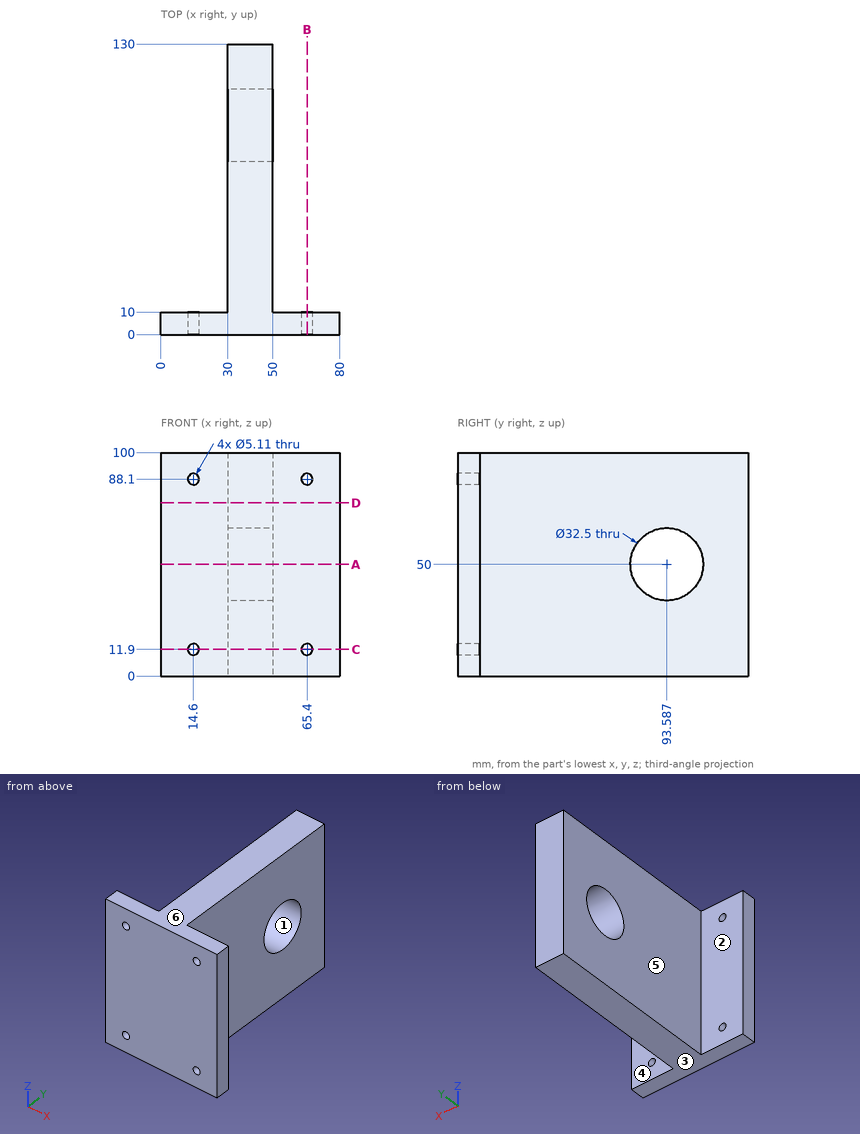
The drawing under review shows one solid part. Ordinate dimensions are in mm from its lowest x, y, z. A direction names the side the tool comes from. Round coordinates to 2 decimals unless told otherwise and drop trailing zeros. Loops run counter-clockwise (first coordinate to the right, second up) from the corner with the lowest first, then second, coordinate; pieces in that order, holes last. Notation, with made-up numbers: (81.5, 80) -> (125.5, 80) arc R11 cw to (125.5, 92) -> close; hole circle Ø8 at (29, 56). An arc over 180 degrees is marked (long way). One line per question, with ' | ' between items. Start each with the question number.
Item 1: For pin 1 (6 mm diameter, centred on y = 57, z = 31.5, fed in from +X); pin 2 (8 mm diameter, centred on x = 12.5, z = 88.5, fed in from +Y), all flat-tipped, find the tip position at first contact; note any pin that passes through.
Item 2: Add section D-D, the plane z = 77.5. Write out the cut boundary in (x, y), then the cut area to 3 significant figures.
Item 3: Wall thickness on line 1 along Z through (x, y) = (14.6, 2.25) (3 decimals); line 2 along Z through (x, y) = (65, 8); line 3 along X through (y, z) = (5, 88): over which ranges is each line inside the solid? List them lowest first. Write a range as [from, to].
Item 4: Add section A-A, the plane z = 50. Write out the cut boundary in (x, y).
Item 5: Draft analysis for pull direction Z (two halves, no side actions). For the marked faces 1, 2 and 3, state which applies: +Z half, -Z half, draft (parallel to the pull), parting line (faces both ways), or undercut.
Item 6: Machinability: for the marked faces 4, 5 and 6, which of the approach directions +Z, -Z, +X, -X, +Y, -Y give a long, thin tool a straight path to every point of the face, cutting with its end or side? Answer none if there is none.
Item 7: Add section C-C, the plane z = 11.9. Write out the cut boundary in (x, y) (3 decimals), then the cut area to 3 significant figures.
Item 8: Add section B-B, the plane x = 65.4. Write out the cut boundary in (y, z) (3 decimals).
Return value:
1) pin 1: stops at x = 50 | pin 2: stops at y = 10
2) outline: (0, 0) -> (80, 0) -> (80, 10) -> (50, 10) -> (50, 130) -> (30, 130) -> (30, 10) -> (0, 10) -> close | area: 3,200 mm2
3) line 1: z = [0, 9.345], [14.455, 85.545], [90.655, 100] | line 2: z = [0, 9.38], [14.42, 85.58], [90.62, 100] | line 3: x = [0, 12.05], [17.15, 62.85], [67.95, 80]
4) outline: (0, 0) -> (80, 0) -> (80, 10) -> (50, 10) -> (50, 77.34) -> (30, 77.34) -> (30, 10) -> (0, 10) -> close; (30, 109.84) -> (50, 109.84) -> (50, 130) -> (30, 130) -> close
5) face 1: undercut | face 2: draft | face 3: -Z half
6) face 4: +Z, -Z, +X, +Y | face 5: +Z, -Z, -X, +Y | face 6: +Z, +X, -X, +Y, -Y
7) outline: (0, 0) -> (12.045, 0) -> (12.045, 10) -> (0, 10) -> close; (17.155, 0) -> (62.845, 0) -> (62.845, 10) -> (50, 10) -> (50, 130) -> (30, 130) -> (30, 10) -> (17.155, 10) -> close; (67.955, 0) -> (80, 0) -> (80, 10) -> (67.955, 10) -> close | area: 3,100 mm2
8) outline: (0, 0) -> (10, 0) -> (10, 9.345) -> (0, 9.345) -> close; (0, 14.455) -> (10, 14.455) -> (10, 85.545) -> (0, 85.545) -> close; (0, 90.655) -> (10, 90.655) -> (10, 100) -> (0, 100) -> close
